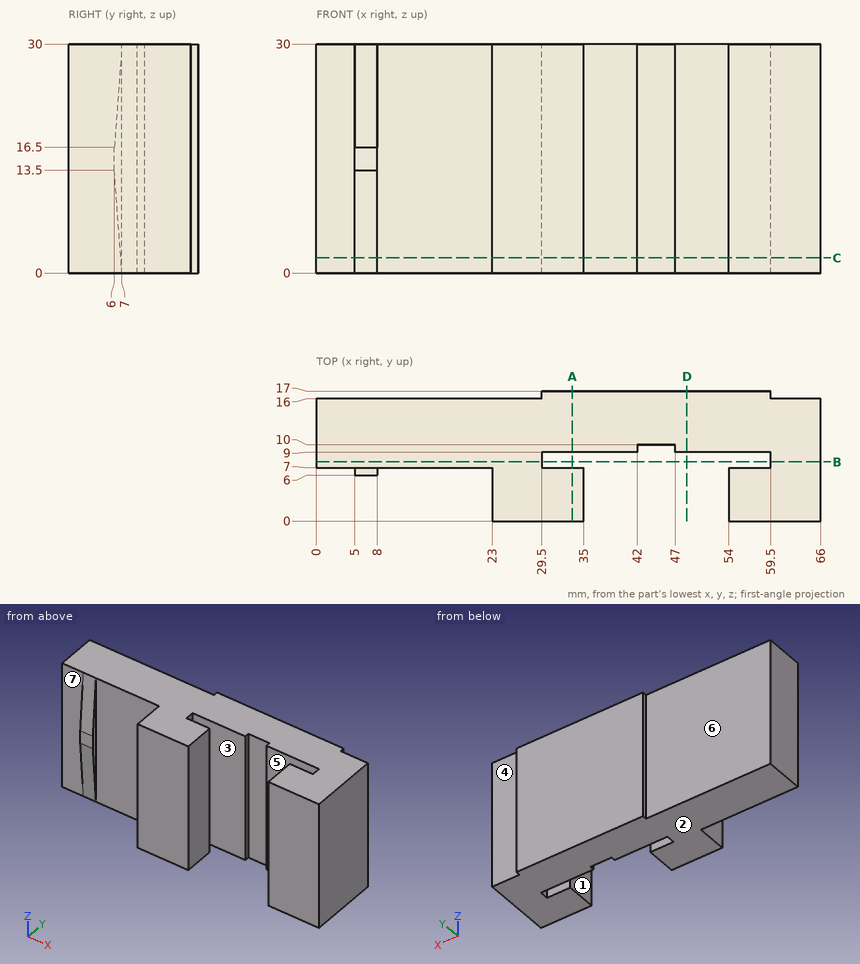
Could you check a few things on this drawing? It's one solid part, dimensions in mm from its lowest x, y, z. A direction names the side the tool comes from. Give positions to 0.01 mm unless a question says otherwise; leave off trailing zeros. Order: outer loops, then holes, each group sorted by start corner. A loop starts at its lowest first (then second) coordinate and runs counter-clockwise, first axis right, second up. Notation, with made-up numbers: M -18,23.5 L 5,23.5 A25 ccw 5,41.5 Z; hole C 23,60 d4. An arc over 180 degrees is marked long. Use one line per item in the form item = value. Start each with the question number.
Item 1: For the marked faces 1, 2, 3 and 4, which set-ups out of +Z, -Z, +X, -X, +Y, -Y let a thin tool reach every point of the face, with its end or its side?
Item 2: If we section it at A-A (x = 33.5): Write out the boundary of the cut face in (y, z), then the cut area to 3 significant figures.
Item 3: If we section it at C-C (z = 2): Write out the boundary of the cut face in (x, y), then the cut area to 3 significant figures.
Item 4: If we section it at B-B (y = 7.75): Write out the boundary of the cut face in (x, z), then the cut area to 3 significant figures.
Item 5: If I drill on line 1 along X through (y, z) = (3.5, 12); line 2 along X through (y, z) = (8.25, 26); line 3 along Y through (x, z) = (25, 5), over which ranges is the centre line in solid material (lowest first)?
Item 6: Will these pins go through, and if not, where does the flat tip stop? pin 1 Ø1.5 at (x, z) = (3.5, 21.5) entering from -Y; pin 2 Ø3 at (x, z) = (43, 9.5) entering from -Y; pin 3 Ø0.5 at (y, z) = (6.5, 16) entering from -X.
Item 7: If we section it at D-D (x = 48.5): Write out the boundary of the cut face in (y, z), then the cut area to 3 significant figures.
Item 8: We'd pull the mould along Y, two halves only. Please class the marked faces 5, 6 and 7: +Y half, -Y half, draft (parallel to the pull), parting line (faces both ways), or undercut.
Outcome:
q1.face_1 = +Z, -Z, -Y
q1.face_2 = -Z, +X, -X, +Y, -Y
q1.face_3 = +Z, -Z
q1.face_4 = +Z, -Z, +X, +Y
q2.outline = M 0,0 L 7,0 L 7,30 L 0,30 Z; M 9,0 L 17,0 L 17,30 L 9,30 Z
q2.area = 450 mm2
q3.outline = M 0,7 L 5,7 L 5,6.85 L 8,6.85 L 8,7 L 23,7 L 23,0 L 35,0 L 35,7 L 29.5,7 L 29.5,9 L 42,9 L 42,10 L 47,10 L 47,9 L 59.5,9 L 59.5,7 L 54,7 L 54,0 L 66,0 L 66,16 L 59.5,16 L 59.5,17 L 29.5,17 L 29.5,16 L 0,16 Z
q3.area = 727 mm2
q4.outline = M 0,0 L 29.5,0 L 29.5,30 L 0,30 Z; M 59.5,0 L 66,0 L 66,30 L 59.5,30 Z
q4.area = 1,080 mm2
q5.line_1 = 23 to 35, 54 to 66
q5.line_2 = 0 to 29.5, 59.5 to 66
q5.line_3 = 0 to 16
q6.pin_1 = 7
q6.pin_2 = 9
q6.pin_3 = 5
q7.outline = M 9,0 L 17,0 L 17,30 L 9,30 Z
q7.area = 240 mm2
q8.face_5 = undercut
q8.face_6 = +Y half
q8.face_7 = -Y half
